from build123d import *

# Parameters (mm, degrees)
BOSS_EXTRUDE1_DEPTH = 8
SKETCH2_R           = 1.5
BOSS_EXTRUDE2_DEPTH = 6
BOSS_EXTRUDE3_DEPTH = 5
SKETCH6_W           = 6.69152868
SKETCH6_H           = 6.205945627
BOSS_EXTRUDE6_DEPTH = 1
SKETCH7_R           = 2.018356376
CUT_EXTRUDE1_DEPTH  = 1


with BuildPart() as part:
    # Sketch1 → Boss-Extrude1 (new body)
    with BuildSketch(Plane.XY):
        with BuildLine():
            Line((-26.903550099, 0), (23.096449901, 0))
            Line((23.096449901, 0), (23.096449901, -0.7))
            ThreePointArc((23.096449901, -0.7), (21.046197369, -5.649747468), (16.096449901, -7.7))
            Line((16.096449901, -7.7), (-19.903550099, -7.7))
            ThreePointArc((-19.903550099, -7.7), (-24.853297568, -5.649747468), (-26.903550099, -0.7))
            Line((-26.903550099, -0.7), (-26.903550099, 0))
        make_face()
    extrude(amount=BOSS_EXTRUDE1_DEPTH)

    # Sketch2 → Boss-Extrude2 (add)
    with BuildSketch(Plane.XY.offset(8)):
        with Locations((-17.076235964, -3.85)):
            Circle(SKETCH2_R)
    extrude(amount=BOSS_EXTRUDE2_DEPTH)

    # Sketch3 → Boss-Extrude3 (add, symmetric)
    with BuildSketch(Plane(origin=(0, 0, 0), x_dir=(0, 0, -1), z_dir=(1, 0, 0))):
        Polygon((-4, -7.7), (-13.024577684, -27.7), (-25.024577684, -27.7), (-27.207163102, -27.7), (-27.207163102, -25.7), (-25.024577684, -25.7), (-15.609285193, -25.7), (-7.487165278, -7.7), align=None)
    extrude(amount=BOSS_EXTRUDE3_DEPTH, both=True)

    # Sketch6 → Boss-Extrude6 (add)
    with BuildSketch(Plane(origin=(0, 1.504350405, 3.333896515), x_dir=(1, 0, 0), z_dir=(0, 0.411295964451016, 0.911501853879798))):
        with Locations((0, -16.088463414)):
            Rectangle(SKETCH6_W, SKETCH6_H)
    extrude(amount=BOSS_EXTRUDE6_DEPTH)

    # Sketch7 → Cut-Extrude1 (cut)
    with BuildSketch(Plane.XY.offset(8)):
        with Locations((-5.657616705, -3.562287369)):
            Circle(SKETCH7_R)
        with Locations((4.040388693, -3.562287369)):
            Circle(SKETCH7_R)
    extrude(amount=-CUT_EXTRUDE1_DEPTH, mode=Mode.SUBTRACT)

    # Sketch10 → Revolve2 (revolve)
    with BuildSketch(Plane(origin=(0, 0, 0), x_dir=(0, 0, -1), z_dir=(1, 0, 0)), mode=Mode.PRIVATE) as revolve2_sk:
        with BuildLine():
            Line((-22.996998778, -25.7), (-21.408224147, -25.7))
            Line((-21.408224147, -25.7), (-21.408224147, -15.873742871))
            add(Edge.make_bspline(
                [(-21.408224147, -15.873742871), (-22.370300932, -16.046682358), (-22.408224147, -16.666364236)],
                knots=[0, 0, 0, 0.92415357, 0.92415357, 0.92415357], degree=2))
            Line((-22.408224147, -16.666364236), (-22.408224147, -16.771089476))
            Line((-22.408224147, -16.771089476), (-22.342150898, -24.712427098))
            ThreePointArc((-22.342150898, -24.712427098), (-22.931989874, -25.03220925), (-22.996998778, -25.7))
        make_face()
    revolve(revolve2_sk.sketch.rotate(Axis((0, -25.7, 21.408224147), (0, 1, 0)), 180), axis=Axis((0, -25.7, 21.408224147), (0, 1, 0)))


solid = part.part
Here's how the part is built. I have some questions about the finished solid (model axes, mm). A direction names the side the tool comes from. Coordinates: 2 decimals unless noted, no trailing zeros. Write each loop counter-clockwise with the first axis right and the second up, starting at its lowest first coordinate (ties: lowest second). Pieces come first, ordered by that corner, then holes.
1) I'm going to push flat-ended pins straight in: pin 1 (6.5 mm diameter, centred on x = 2.5, z = 4, fed in from -Y); pin 2 (6 mm diameter, centred on x = -4.5, y = -2, fed in from +Z); pin 3 (2 mm diameter, centred on x = -18, z = 8, fed in from -Y); pin 4 (2.5 mm diameter, centred on x = -5.66, y = -3.56, fed in from -Z). Where does each tip first touch, or does it pass through?
Filled in:
pin 1: stops at y = -14.9
pin 2: stops at z = 8
pin 3: stops at y = -7.7
pin 4: stops at z = 0
2) If I drill on line 1 (Y direction, x = -3.5, z = 20.5); line 2 (Z direction, x = 21, y = -2.5); line 3 (X direction, y = -12.75, z = 10), over which ranges is the centre line in solid material (lowest first)?
Filled in:
line 1: y = -27.7 to -25.7
line 2: z = 0 to 8
line 3: x = -3.35 to 3.35
3) Which directions (+Z, -Z, +X, -X, +Y, -Y) give clear straight access to the entire face, cutting with the end or side of a thin tool? Please do faces 1 (the face through (-6, -4, 7)), 2 (the face through (5, -20, 12)), 3 (the face through (-17, -4, 14)), 4 (the face through (-0.29, -20.797, 20.486)), 5 (the face through (3.346, -13, 10.4)).
Filled in:
face 1: +Z
face 2: +Z, -Z, +X, -Y
face 3: +Z, +X, -X, +Y, -Y
face 4: none
face 5: +Z, +X, +Y
4) If we section it at D-D (y = -21): List the corners of the cut face in (x, z) for me, plus the area to 3 significant figures.
Filled in:
outline: (-5, 10) - (5, 10) - (5, 13.49) - (-5, 13.49) - close; circle Ø1.93 at (0, 21.41)
area: 37.8 mm2
5) Thinking about a two-plate mould opening in Z: for faces 6 (the face through (0, -27, 27.207)), 7 (the face through (1.2, -25.7, 20)), 8 (the face through (0, -27.7, 20)), which applies, +Z half, -Z half, draft (parallel to the pull), parting line (faces both ways), or undercut?
Filled in:
face 6: +Z half
face 7: undercut
face 8: draft
6) If we section it at C-C (x = 9.5): List the corners of the cut face in (y, z) for me.
Filled in:
outline: (-7.7, 0) - (0, 0) - (0, 8) - (-7.7, 8) - close
7) If we section it at A-A (z = 2.75): List the corners of the cut face in (x, y) for me, plus the area to 3 significant figures.
Filled in:
outline: (-26.9, -0.7) arc R7 ccw to (-19.9, -7.7) - (16.1, -7.7) arc R7 ccw to (23.1, -0.7) - (23.1, 0) - (-26.9, 0) - close
area: 364 mm2
8) If we section it at B-B (y = -13): List the corners of the cut face in (x, z) for me.
Filled in:
outline: (-5, 6.39) - (5, 6.39) - (5, 9.88) - (3.35, 9.88) - (3.35, 10.98) - (-3.35, 10.98) - (-3.35, 9.88) - (-5, 9.88) - close
